Could you check a few things on this model? Use its own coordinates, in mm. Coordinates: 2 decimals unless noted, no trailing zeros. Write each loop counter-clockwise with the first axis right and the second up, starting at its lowest first coordinate (ties: lowest second). Pieces come first, ordered by that corner, then holes.
```python
from build123d import *

# Parameters (mm, degrees)
SKETCH_1_W         = 300
SKETCH_1_H         = 140
EXTRUDE_1_DEPTH    = 1
HOLE_WIZARD_M5_1_D = 5.5


with BuildPart() as part:
    # 스케치1 → 보스-돌출1 (new body)
    with BuildSketch(Plane.XY):
        Rectangle(SKETCH_1_W, SKETCH_1_H)
    extrude(amount=EXTRUDE_1_DEPTH)

    # M5 여유 구멍1 (through all)
    with Locations(Plane(origin=(0, 0, 0), x_dir=(-1, 0, 0), z_dir=(0, 0, -1))):
        with Locations((-140, 60), (-70, 60), (70, 60), (0, 60), (140, 60), (140, 0), (140, -60), (-140, 0), (-140, -60), (-70, -60), (70, -60), (0, -60)):
            Hole(HOLE_WIZARD_M5_1_D / 2)


solid = part.part
```
1. I want a section at B-B on y = -60. Please give me the cut outline in (x, z).
Verdict:
outline: (-150, 0) - (-142.75, 0) - (-142.75, 1) - (-150, 1) - close; (-137.25, 0) - (-72.75, 0) - (-72.75, 1) - (-137.25, 1) - close; (-67.25, 0) - (-2.75, 0) - (-2.75, 1) - (-67.25, 1) - close; (2.75, 0) - (67.25, 0) - (67.25, 1) - (2.75, 1) - close; (72.75, 0) - (137.25, 0) - (137.25, 1) - (72.75, 1) - close; (142.75, 0) - (150, 0) - (150, 1) - (142.75, 1) - close
2. If we mould it in two halves opening along X, with no side actions, what happens to faces 1 (the face through (141.48, 62.32, 0.51)), 2 (the face through (-138.52, -57.68, 0.51)), 3 (the face through (-2, 1, 0))? For each: pulls with the +X half, pulls with the -X half, needs draft (parallel to the pull), parting line crosses it, or undercut.
Verdict:
face 1: undercut
face 2: undercut
face 3: needs draft
3. I want a section at D-D on y = 0. Please give me the cut outline in (x, z), plus the area to 3 significant figures.
Verdict:
outline: (-150, 0) - (-142.75, 0) - (-142.75, 1) - (-150, 1) - close; (-137.25, 0) - (137.25, 0) - (137.25, 1) - (-137.25, 1) - close; (142.75, 0) - (150, 0) - (150, 1) - (142.75, 1) - close
area: 289 mm2
4. I want a section at C-C on x = -70. Please give me the cut outline in (y, z), plus the area to 3 significant figures.
Verdict:
outline: (-70, 0) - (-62.75, 0) - (-62.75, 1) - (-70, 1) - close; (-57.25, 0) - (57.25, 0) - (57.25, 1) - (-57.25, 1) - close; (62.75, 0) - (70, 0) - (70, 1) - (62.75, 1) - close
area: 129 mm2
5. I want a section at A-A on x = 140. Please give me the cut outline in (y, z), plus the area to 4 significant figures.
Verdict:
outline: (-70, 0) - (-62.75, 0) - (-62.75, 1) - (-70, 1) - close; (-57.25, 0) - (-2.75, 0) - (-2.75, 1) - (-57.25, 1) - close; (2.75, 0) - (57.25, 0) - (57.25, 1) - (2.75, 1) - close; (62.75, 0) - (70, 0) - (70, 1) - (62.75, 1) - close
area: 123.5 mm2
6. Please list where these lines run through material, in increasing order: line 1 along Y through (x, z) = (-70, 0.3); line 2 along Y through (x, z) = (-140, 0.6); line 3 along X through (y, z) = (-1.5, 0.7).
Verdict:
line 1: y = -70 to -62.75, -57.25 to 57.25, 62.75 to 70
line 2: y = -70 to -62.75, -57.25 to -2.75, 2.75 to 57.25, 62.75 to 70
line 3: x = -150 to -142.3, -137.7 to 137.7, 142.3 to 150
